Check sheet for the modelled part. Datum: model origin and axes. Units: mm. A direction names the side the tool comes from. Round coordinates to 2 decimals unless told otherwise and drop trailing zeros. Write each loop counter-clockwise with the first axis right and the second up, starting at its lowest first coordinate (ties: lowest second). Pieces come first, ordered by that corner, then holes. Notation, with made-up numbers: M -30.5,59.25 L 20.5,59.25 A11 cw 20.5,77.25 Z; hole C 72.25,41 d2. An arc over 180 degrees is marked long. One line per item, written item: value.
from build123d import *

# Parameters (mm, degrees)
F0_W          = 23
F0_H          = 6
F1_DEPTH      = 11
F2_W          = 3.8415808491
F2_H          = 9.9605580419
F2_R          = 1.5
F3_DEPTH      = 4
F4_DEPTH      = 6
F5_T1_DEPTH   = 9
F6_W          = 23
F6_H          = 6
F6_W_2        = 17
F7_DEPTH      = 4.5
F8_W          = 12
F8_H          = 4.5
F8_W_2        = 5
F9_DEPTH      = 25
F11_DEPTH     = 3
F12_W         = 15
F12_H         = 25
F12_W_2       = 4.5
F13_DEPTH     = 4.5
F14_T1_DEPTH  = 6
F14_T3_DEPTH  = 49.8746859277
F14_T5_DEPTH  = 37.5
F14_T7_DEPTH  = 37.4373429638
F14_T9_DEPTH  = 31
F14_T11_DEPTH = 31
F14_T13_DEPTH = 31


# Not quite as in the source:
# - a fillet or chamfer that OpenCascade refuses, or shapes differently, is made with other operations: its cross-section is extruded or revolved along the edge and cut away or added


with BuildPart() as f1:
    # F0 (on Front) → F1 (new body)
    with BuildSketch(Plane.XZ):
        Rectangle(F0_W, F0_H)
    extrude(amount=-F1_DEPTH)

    # F2 (on face) → F3 (join)
    with BuildSketch(Plane.XY.offset(3)):
        with Locations((6.5, 5)):
            Rectangle(F2_W, F2_H)
        with Locations((6.5, 5)):
            Circle(F2_R, mode=Mode.SUBTRACT)
    extrude(amount=F3_DEPTH)

    # F4 (cut): a face of the model
    f4_faces = [f1.faces().sort_by_distance(p)[0] for p in [
        (6.5, 5, 3),
    ]]
    extrude(f4_faces, amount=-F4_DEPTH, mode=Mode.SUBTRACT)

    # F5: fillet of radius 2 on 2 edges, made by hand

    # F5_s2 → F5_t1 (cut)
    with BuildSketch(Plane.XY.offset(3)):
        with BuildLine():
            ThreePointArc((6.4207904246, 0.019720979), (7.8350039869, 0.6055074167), (8.4207904246, 2.019720979))
            Line((8.4207904246, 2.019720979), (8.4207904246, 0.019720979))
            Line((8.4207904246, 0.019720979), (6.4207904246, 0.019720979))
        make_face()
        with BuildLine():
            ThreePointArc((4.5792095754, 2.019720979), (5.1649960131, 0.6055074167), (6.5792095754, 0.019720979))
            Line((6.5792095754, 0.019720979), (4.5792095754, 0.019720979))
            Line((4.5792095754, 0.019720979), (4.5792095754, 2.019720979))
        make_face()
    extrude(amount=F5_T1_DEPTH, mode=Mode.SUBTRACT)

    # F6 (on face) → F7 (join)
    with BuildSketch(Plane(origin=(0, 11, 0), x_dir=(-1, 0, 0), z_dir=(0, 1, 0))):
        Rectangle(F6_W, F6_H)
        with Locations((20, 0)):
            Rectangle(F6_W_2, F6_H)
    extrude(amount=F7_DEPTH)

    # F8 (on face) → F9 (join)
    with BuildSketch(Plane.XY.offset(3)):
        with Locations((-17.5, 13.25)):
            Rectangle(F8_W, F8_H)
        with Locations((-9, 13.25)):
            Rectangle(F8_W_2, F8_H)
    extrude(amount=F9_DEPTH)

    # F10 (on face) → F11 (join)
    with BuildSketch(Plane(origin=(0, 15.5, 0), x_dir=(-1, 0, 0), z_dir=(0, 1, 0))):
        Polygon((6.5, 3), (-11.5, 3), (-11.5, -3), (28.5, -3), (28.5, 3), (23.5, 3), align=None)
    extrude(amount=F11_DEPTH)

    # F12 (on face) → F13 (join)
    with BuildSketch(Plane.YZ.offset(-6.5)):
        with Locations((23, 15.5)):
            Rectangle(F12_W, F12_H)
        with Locations((13.25, 15.5)):
            Rectangle(F12_W_2, F12_H)
    extrude(amount=F13_DEPTH)

    # F14: fillet of radius 5 on 7 edges, made by hand

    # F14_s2 → F14_t1 (join)
    with BuildSketch(Plane.XY.offset(-3)):
        with BuildLine():
            ThreePointArc((-16.5, 11), (-12.9644660941, 9.5355339059), (-11.5, 6))
            Line((-11.5, 6), (-11.5, 11))
            Line((-11.5, 11), (-16.5, 11))
        make_face()
    extrude(amount=F14_T1_DEPTH)

    # F14_s4 → F14_t3 (cut)
    with BuildSketch(Plane.XY.offset(-9.4373429638)):
        with BuildLine():
            ThreePointArc((-2, 25.5250628145), (-3.2919007565, 28.8791647807), (-6.5, 30.5))
            Line((-6.5, 30.5), (-2, 30.5))
            Line((-2, 30.5), (-2, 25.5250628145))
        make_face()
    extrude(amount=F14_T3_DEPTH, mode=Mode.SUBTRACT)

    # F14_s6 → F14_t5 (cut)
    with BuildSketch(Plane.XY.offset(3)):
        with BuildLine():
            ThreePointArc((-7, 11), (-3.4644660941, 12.4644660941), (-2, 16))
            Line((-2, 16), (-2, 11))
            Line((-2, 11), (-7, 11))
        make_face()
    extrude(amount=F14_T5_DEPTH, mode=Mode.SUBTRACT)

    # F14_s8 → F14_t7 (cut)
    with BuildSketch(Plane.XY.offset(3)):
        with BuildLine():
            ThreePointArc((-18.5250628145, 11), (-21.8791647807, 12.2919007565), (-23.5, 15.5))
            Line((-23.5, 15.5), (-23.5, 11))
            Line((-23.5, 11), (-18.5250628145, 11))
        make_face()
    extrude(amount=F14_T7_DEPTH, mode=Mode.SUBTRACT)

    # F14_s10 → F14_t9 (cut)
    with BuildSketch(Plane.XY.offset(-15.5)):
        with BuildLine():
            ThreePointArc((11.5, 5), (10.0355339059, 1.4644660941), (6.5, 0))
            Line((6.5, 0), (11.5, 0))
            Line((11.5, 0), (11.5, 5))
        make_face()
    extrude(amount=F14_T9_DEPTH, mode=Mode.SUBTRACT)

    # F14_s12 → F14_t11 (cut)
    with BuildSketch(Plane.XY.offset(-15.5)):
        with BuildLine():
            ThreePointArc((-6.5, 0), (-10.0355339059, 1.4644660941), (-11.5, 5))
            Line((-11.5, 5), (-11.5, 0))
            Line((-11.5, 0), (-6.5, 0))
        make_face()
    extrude(amount=F14_T11_DEPTH, mode=Mode.SUBTRACT)

    # F14_s14 → F14_t13 (cut)
    with BuildSketch(Plane.XY.offset(-15.5)):
        with BuildLine():
            ThreePointArc((-28.5, 16), (-27.0355339059, 12.4644660941), (-23.5, 11))
            Line((-23.5, 11), (-28.5, 11))
            Line((-28.5, 11), (-28.5, 16))
        make_face()
    extrude(amount=F14_T13_DEPTH, mode=Mode.SUBTRACT)


solid = f1.part
Q1. Scan lines: line 1 (Y direction, x = 6.5, z = -0.7); line 2 (X direction, y = 24, z = 15); line 3 (Y direction, x = 6.5, z = 5.55). Record each from-to range of solid material in increasing order. Write a range as [from, to].
Completed:
line 1: [0, 3.5], [6.5, 18.5]
line 2: [-6.5, -2]
line 3: [0.02, 3.5], [6.5, 9.98]
Q2. Depth check by flat-ended pin: P1, Ø1.5, axis at x = -24.5, z = 24.5, coming from the +Y side; P2, Ø4.5, axis at y = 22.5, z = 16, coming from the -X side; P3, Ø13.5, axis at x = -12, z = 21.5, coming from the +Y side; P4, Ø4, axis at x = 7, y = 3, coming from the +Z side. Enter the tip coordinate at first touch or a pass-through.
Completed:
P1: through
P2: x = -6.5
P3: y = 30.5
P4: z = 7
Q3. Sectioned sample at C-C on y = 9. Enter the section's corners in (x, z).
Completed:
outline: M -12.5,-3 L 11.5,-3 L 11.5,3 L 8.42,3 L 8.42,7 L 4.58,7 L 4.58,3 L -12.5,3 Z
Q4. Sectioned sample at B-B on z = 1. Enter the section's corners in (x, y), and give its area (3 significant figures).
Completed:
outline: M -28.5,16 A5 ccw -23.5,11 L -16.5,11 A5 cw -11.5,6 L -11.5,5 A5 ccw -6.5,0 L 6.5,0 A5 ccw 11.5,5 L 11.5,18.5 L -28.5,18.5 Z; hole C 6.5,5 d3
area: 535 mm^2
Q5. Access from +Z, -Z, +X, -X, +Y, -Y to the whole of each face (thin tool, end or side, straight path). Record for faces 1 (the flat face through (4.579, 6, 5)), 2 (the flat face through (6, 9.98, 5)), 3 (the flat face through (-14, 11, 12)), 4 (the flat face through (8.421, 6, 5)).
Completed:
face 1: +Z, -X, +Y, -Y
face 2: +Z, +X, -X, +Y
face 3: +Z, -X, -Y
face 4: +Z, +X, +Y, -Y
Q6. Sectioned sample at A-A on y = 4.5. Enter the section's corners in (x, z).
Completed:
outline: M -11.47,-3 L 5.09,-3 L 5.09,7 L 4.58,7 L 4.58,3 L -11.47,3 Z; M 7.91,-3 L 11.47,-3 L 11.47,3 L 8.42,3 L 8.42,7 L 7.91,7 Z
Q7. Sectioned sample at D-D on z = 9.5. Enter the section's corners in (x, y).
Completed:
outline: M -23.5,15.5 A5 ccw -18.53,11 L -7,11 A5 ccw -2,16 L -2,25.53 A5 ccw -6.5,30.5 L -6.5,15.5 Z
